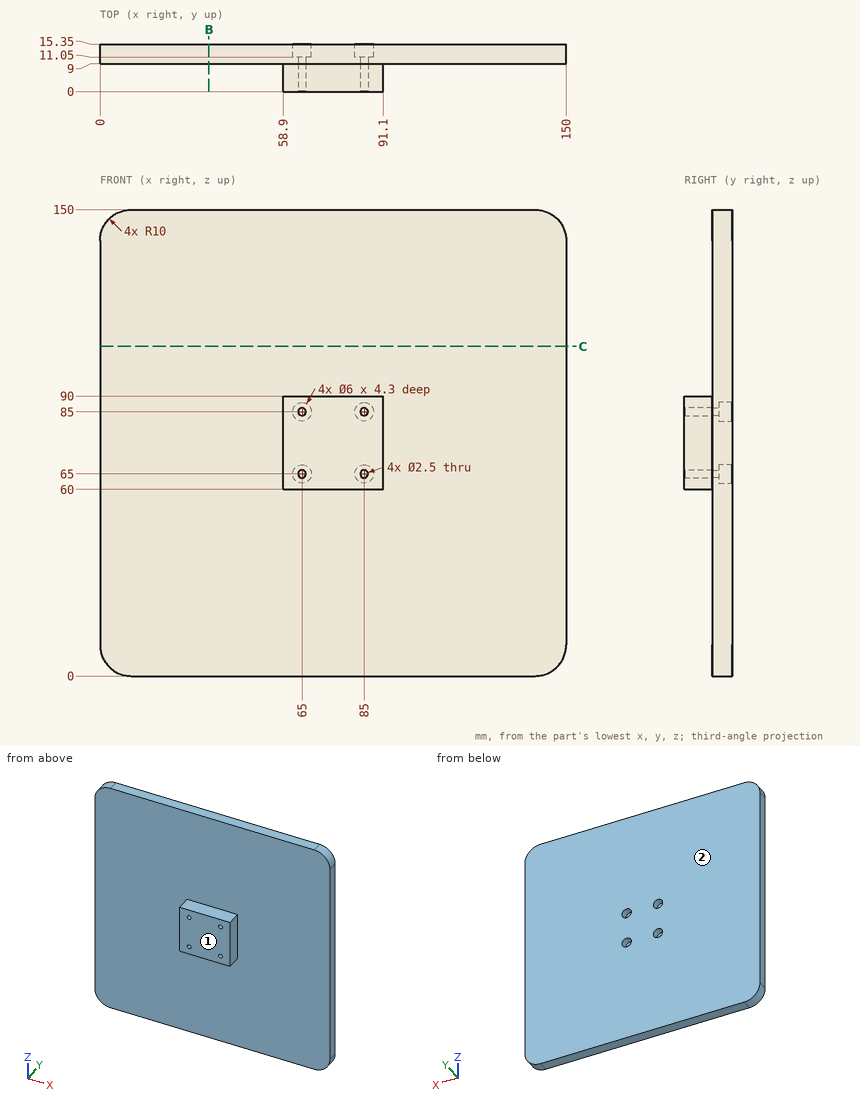
Input: dimensioned drawing with shaded views. Units: mm. Origin: part minimum x, y, z. Coordinates: 2 decimals unless noted, no trailing zeros. Order: outer loops, then holes, each group sorted by start corner. A loop starts at its lowest first (then second) coordinate and runs counter-clockwise, first axis right, second up. Notation, with made-up numbers: (4, -24.5) -> (12, -24.5) arc R10 ccw to (12, -15.5) -> close; hole circle Ø7 at (39.25, 88.5). An arc over 180 degrees is marked (long way). Answer in a Markdown table with one row per item.
Item 1: Section B-B on x = 35. Output: boundary loops of the cut face in (y, z).
Return value:
| item | result |
|---|---|
| outline | (9, 0) -> (15.35, 0) -> (15.35, 150) -> (9, 150) -> close |
Item 2: Contact query for flat-ended pins moving along their axis: P1, Ø6, axis at x = 25, z = 75, coming from the -Y side; P2, Ø2, axis at x = 65, z = 85, coming from the +Y side; P3, Ø3, axis at x = 85, z = 85, coming from the +Y side; P4, Ø4.5, axis at x = 76.5, y = 2.5, coming from the -Z side. Output: stop coordinate, or through.
Return value:
| item | result |
|---|---|
| P1 | stops at y = 9 |
| P2 | passes through |
| P3 | stops at y = 11.05 |
| P4 | stops at z = 60 |
Item 3: Section C-C on z = 106. Output: boundary loops of the cut face in (x, y), plus the area to 4 significant figures.
Return value:
| item | result |
|---|---|
| outline | (0, 9) -> (150, 9) -> (150, 15.35) -> (0, 15.35) -> close |
| area | 952.5 mm² |
Item 4: Draft query along Y for the marked faces 1 and 2. Return one class per face: released by +Y, released by -Y, zero draft, split by the parting line, or undercut.
Return value:
| item | result |
|---|---|
| face 1 | released by -Y |
| face 2 | released by +Y |
Item 5: Ray query, L1, parallel to X at y = 5.5, z = 85; L2, parallel to Z at x = 85, y = 6.25; L3, parallel to Z at x = 65, y = 9.85. Return the intervals inside material, ascending.
Return value:
| item | result |
|---|---|
| L1 | x = 58.9 to 63.75, 66.25 to 83.75, 86.25 to 91.1 |
| L2 | z = 60 to 63.75, 66.25 to 83.75, 86.25 to 90 |
| L3 | z = 0 to 63.75, 66.25 to 83.75, 86.25 to 150 |
